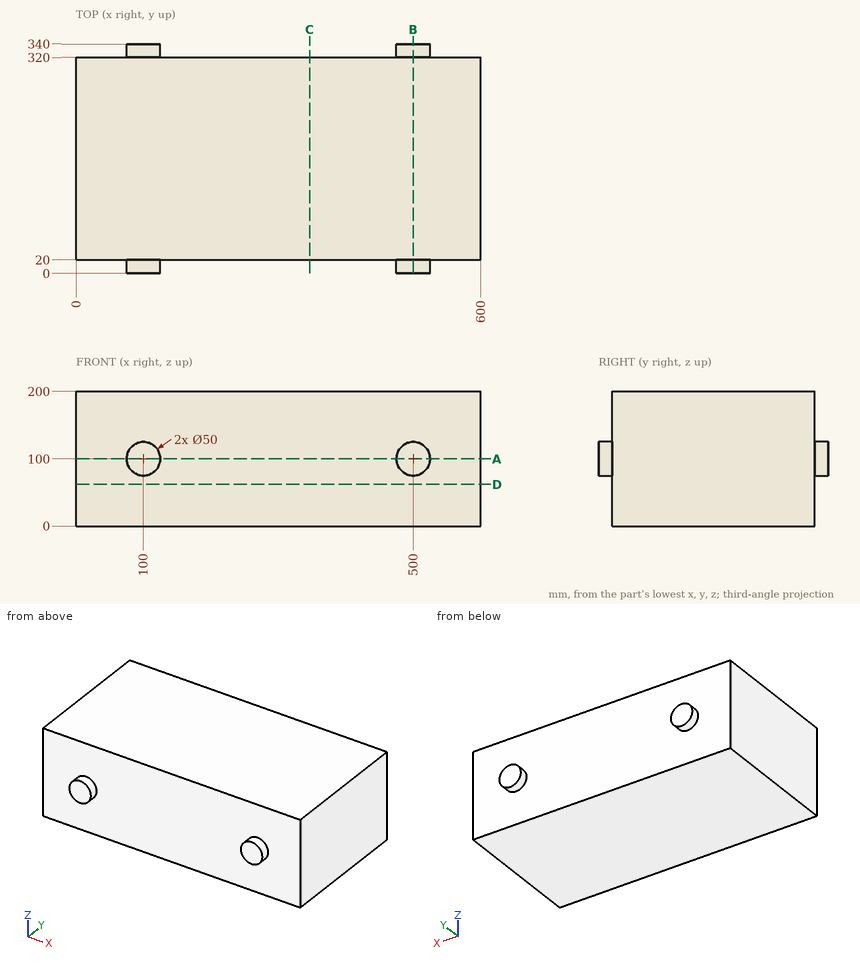
Source: three-view drawing plus pictorial views. Frame: mm from the lowest corner of the part. Coordinates: 2 decimals unless noted, no trailing zeros. Order: outer loops, then holes, each group sorted by start corner. A loop starts at its lowest first (then second) coordinate and runs counter-clockwise, first axis right, second up. Notation, with made-up numbers: M 35.5,30.25 L 87.5,30.25 A30 ccw 87.5,65.25 Z; hole C -20,6 d8. An arc over 180 degrees is marked long. Write each question's results on one line, items separated by ' | '. Start each with the question number.
1. Material intervals for L1, parallel to Y at x = 110.5, z = 56, sorted ascending.
2. Pin query (flat end, axial travel): pin 1 (1 mm diameter, centred on x = 375, z = 165, fed in from +Y); pin 2 (10 mm diameter, centred on x = 449, z = 168, fed in from -Y); pin 3 (8 mm diameter, centred on y = 188.5, z = 99.5, fed in from -X). Return the tip coordinate at first contact, or that it passes through.
3. Section B-B, the plane x = 500. Return the cut outline in (y, z).
4. Section D-D, the plane z = 62. Return the cut outline in (x, y), then the cut area to 3 significant figures.
5. Section A-A, the plane z = 100. Return the cut outline in (x, y).
6. Section C-C, the plane x = 346.5. Return the cut outline in (y, z), then the cut area to 3 significant figures.
Solution:
1) L1: 20 to 320
2) pin 1: y = 320 | pin 2: y = 20 | pin 3: x = 0
3) outline: M 0,75 L 20,75 L 20,0 L 320,0 L 320,75 L 340,75 L 340,125 L 320,125 L 320,200 L 20,200 L 20,125 L 0,125 Z
4) outline: M 0,20 L 600,20 L 600,320 L 0,320 Z | area: 180,000 mm²
5) outline: M 0,20 L 75,20 L 75,0 L 125,0 L 125,20 L 475,20 L 475,0 L 525,0 L 525,20 L 600,20 L 600,320 L 525,320 L 525,340 L 475,340 L 475,320 L 125,320 L 125,340 L 75,340 L 75,320 L 0,320 Z
6) outline: M 20,0 L 320,0 L 320,200 L 20,200 Z | area: 60,000 mm²
